Answer from the drawing. Dimensions are ordinates in mm from the lowest x, y and z of the part. A direction names the side the tool comes from. Give positions to 0.01 mm unless a question says otherwise; leave off trailing zeros. Write each loop counter-clockwise with the first axis right and the second up, starting at its lowest first coordinate (ties: lowest second). Pieces come first, ordered by that corner, then holes. Notation, with made-up numbers: (69.25, 43.5) -> (112.25, 43.5) arc R37 ccw to (112.25, 80.5) -> close; hole circle Ø10 at (31.25, -28). An arc over 180 degrees is marked (long way). Write item = value, one per line.
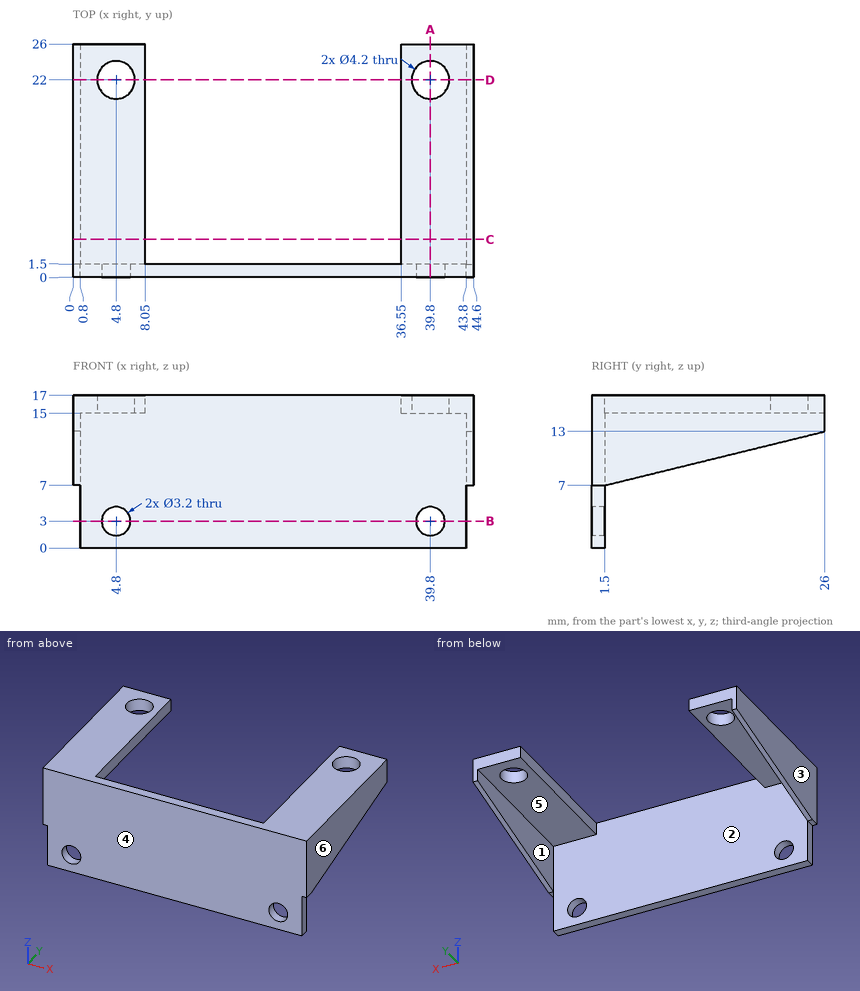
(1) A tool of negligible diameter and unlimited length cuts with its end or side. For the marked faces 5 and 6, from which of +Z, -Z, +X, -X, +Y, -Y can it reach the whole face along a straight path? Write none if from no direction.
Checks:
face_5 = -Z, +Y
face_6 = +Z, -Z, +X, +Y, -Y
(2) The part is cut by section A-A on x = 39.8. Determine the outline of the cut face in (y, z).
Checks:
outline = (0, 0) -> (1.5, 0) -> (1.5, 1.4) -> (0, 1.4) -> close; (0, 4.6) -> (1.5, 4.6) -> (1.5, 15) -> (19.9, 15) -> (19.9, 17) -> (0, 17) -> close; (24.1, 15) -> (26, 15) -> (26, 17) -> (24.1, 17) -> close
(3) For a pull along X with two mould halves and no side action, classify the marked faces 1, 2, 3 and 4 as released by +X, released by -X, zero draft, split by the parting line, or undercut.
Checks:
face_1 = undercut
face_2 = undercut
face_3 = released by -X
face_4 = zero draft
(4) The part is cut by section C-C on y = 4.25. Determine the outline of the cut face in (x, z), plus the area to 3 significant figures.
Checks:
outline = (0, 7.67) -> (0.8, 7.67) -> (0.8, 15) -> (8.05, 15) -> (8.05, 17) -> (0, 17) -> close; (36.55, 15) -> (43.8, 15) -> (43.8, 7.67) -> (44.6, 7.67) -> (44.6, 17) -> (36.55, 17) -> close
area = 43.9 mm²
(5) The part is cut by section B-B on z = 3. Determine the outline of the cut face in (x, y).
Checks:
outline = (0.8, 0) -> (3.2, 0) -> (3.2, 1.5) -> (0.8, 1.5) -> close; (6.4, 0) -> (38.2, 0) -> (38.2, 1.5) -> (6.4, 1.5) -> close; (41.4, 0) -> (43.8, 0) -> (43.8, 1.5) -> (41.4, 1.5) -> close
(6) Consider L1, parallel to X at y = 0.55, z = 3; L2, parallel to Y at x = 39.8, z = 15.5; L3, parallel to Z at x = 39.8, y = 1.05. Determine where each line is inside the solid, lowest interval first.
Checks:
L1 = 0.8 to 3.2, 6.4 to 38.2, 41.4 to 43.8
L2 = 0 to 19.9, 24.1 to 26
L3 = 0 to 1.4, 4.6 to 17
(7) Given P1, Ø4, axis at x = 27.5, z = 11, coming from the +Y side; P2, Ø5.5, axis at x = 39.8, y = 22, coming from the -Z side; P3, Ø1.6, axis at y = 0.5, z = 3, coming from the -X side, each flat-ended and moving along its own axis, determine where each tip first touches the part or whether it passes through.
Checks:
P1 = 1.5
P2 = 15
P3 = 0.8
(8) The part is cut by section D-D on y = 22. Determine the outline of the cut face in (x, z), plus the area to 3 significant figures.
Checks:
outline = (0, 12.02) -> (0.8, 12.02) -> (0.8, 15) -> (2.7, 15) -> (2.7, 17) -> (0, 17) -> close; (6.9, 15) -> (8.05, 15) -> (8.05, 17) -> (6.9, 17) -> close; (36.55, 15) -> (37.7, 15) -> (37.7, 17) -> (36.55, 17) -> close; (41.9, 15) -> (43.8, 15) -> (43.8, 12.02) -> (44.6, 12.02) -> (44.6, 17) -> (41.9, 17) -> close
area = 20.2 mm²
